Read the model definition and answer for the solid it produces. Units are mm, in the model's axes. A direction names the side the tool comes from. Round coordinates to 2 decimals unless told otherwise and drop trailing zeros. Write each loop counter-clockwise with the first axis right and the second up, starting at its lowest first coordinate (ties: lowest second). Pieces come first, ordered by that corner, then holes. Notation, with made-up numbers: (26, 78) - (36, 78) arc R28 cw to (36, 107) - close; hole circle Ø9 at (87.5, 5). An arc over 180 degrees is marked (long way). Answer as CSV lines item,"result". Start each with the question number.
1) Find section B-B on y = 0.45. State how many separate pieces and enclosed holes the cut face has, then the cut area to 3 significant figures.
2) For a pull along Z with two mould halves and no side action, classify faces 3 (the cylindrical face through (-2.216, 1.479, 4.057)), 4 (the flat face through (-5, 3, -23)), 5 (the cylindrical face through (-18.63, 1.48, -22.74)) as +Z half, -Z half, draft (parallel to the pull), parting line (faces both ways), or undercut.
3) Each of these flat-tipped pins is pushed along its axis until it touches: pin 1 (1.5 mm diameter, centred on y = 2, z = -57, fed in from +X) (3 decimals); pin 2 (0.9 mm diameter, centred on y = 1.5, z = -17.5, fed in from -X); pin 3 (1.5 mm diameter, centred on y = 2.5, z = -23, fed in from -X); pin 4 (1.8 mm diameter, centred on x = -9.95, z = -58.27, fed in from +Y). Where does it stop, or does it pass through?
4) Find section C-C on z = -35. Determine the outline of the cut face in (x, y).
5) Find section A-A on x = -5.5. Determine the outline of the cut face in (y, z).
6) Which of the six approach directions +Z, -Z, +X, -X, +Y, -Y give full straight-line access (tool end or side, diameter ignored) to faces 1 (the flat face through (-5, 0, -23)), 2 (the flat face through (-14.361, 1, -18))?
7) Consider line 1 along Z through (x, y) = (-6.75, 2.3); line 2 along Z through (x, y) = (-6.5, 2); line 3 along X through (y, z) = (1.1, -18.5). Determine where each line is inside the solid, lowest interval first.
8) Find section D-D on x = -16. Determine the outline of the cut face in (y, z), then the cut area to 3 significant figures.
Autodesk Inventor part; units mm, degrees
ref_plane "YZ Plane" through (0, 0, 0) normal (1, 0, 0) x (0, 1, 0)
ref_plane "XZ Plane" through (0, 0, 0) normal (0, 1, 0) x (-1, 0, 0)
ref_plane "XY Plane" through (0, 0, 0) normal (0, 0, 1) x (1, 0, 0)
sketch "Sketch1" plane through (0, 0, 0) normal (0, 1, 0) x (-1, 0, 0)
  arc A0 (13.7652, 13.7563) -> (-7.6488, 8.7996) centre (2.9529, 11.7331) ccw
  arc A1 (-7.6488, -55.3335) -> (13.7652, -60.2902) centre (2.9529, -58.2669) ccw
  arc A2 (-7.6723, -55.4199) -> (-7.6723, 8.8861) centre (-125.5725, -23.2669) ccw
  circle A3 centre (2.9529, 11.7331) radius 4.5
  circle A4 centre (2.9529, -58.2669) radius 4.5
  circle A5 centre (2.9529, 4.7331) radius 1
  circle A6 centre (9.9529, 11.7331) radius 1
  circle A7 centre (2.9529, 18.7331) radius 1
  circle A8 centre (-4.0471, 11.7331) radius 1
  circle A9 centre (2.9529, -65.2669) radius 1
  circle A10 centre (9.9529, -58.2669) radius 1
  circle A11 centre (2.9529, -51.2669) radius 1
  circle A12 centre (-4.0471, -58.2669) radius 1
  line L0 (14.3609, -16.1054) -> (10.3609, -16.1054)
  line L1 (10.3609, -16.1054) -> (10.3609, -19.1054)
  line L2 (10.3609, -19.1054) -> (14.3609, -19.1054)
  line L3 (14.3609, -19.1054) -> (14.3609, -16.1054)
  line L4 (14.3609, -11.7669) -> (10.3609, -14.7669) construction
  line L5 (10.3609, -11.7669) -> (14.3609, -14.7669) construction
  line L6 (0.5448, -16.1054) -> (4.5448, -16.1054)
  line L7 (4.5448, -16.1054) -> (4.5448, -19.1054)
  line L8 (4.5448, -19.1054) -> (0.5448, -19.1054)
  line L9 (0.5448, -19.1054) -> (0.5448, -16.1054)
  arc A13 (13.7652, -60.2902) -> (13.7652, 13.7563) centre (-124.6252, -23.2669) ccw
  line L10 (12.3609, -13.2669) -> (12.3609, -13.2669)
  line L11 (10.3609, -18.6054) -> (4.5448, -18.6054)
  line L12 (7.4529, -18.6054) -> (7.4529, -17.6054)
  point P0 (0, 0)
  dimension "d0" = 22
  dimension "d1" = 22
  dimension "d2" = 70
  dimension "d3" = 9
  dimension "d4" = 9
  dimension "d6" = 2
  dimension "d9" = 360
  dimension "d13" = 2
  dimension "d16" = 360
  dimension "d21" = 4
  dimension "d22" = 3
  dimension "d26" = 5.8161
  dimension "d27" = 13.8161
  dimension "d28" = 0
  dimension "d30" = 1
extrude "Extrusion1" add sketch "Sketch1" along normal blind 3
sketch "Sketch2" plane through (0, 3, 0) normal (0, 1, 0) x (1, 0, 0)
  point P0 (0, 0)
sketch "Sketch3" plane through (0, 3, 0) normal (0, 1, 0) x (1, 0, 0)
  point P0 (0, 0)
properties part number "fem"
Check values:
1,separate pieces,"1"
1,enclosed holes,"12"
1,area,"1,760 mm^2"
2,face 3,"undercut"
2,face 4,"draft"
2,face 5,"parting line"
3,pin 1,"stops at x = 8.035"
3,pin 2,"stops at x = -18.53"
3,pin 3,"stops at x = -18.63"
3,pin 4,"passes through"
4,outline,"(-18.15, 0) - (3.93, 0) - (3.93, 3) - (-18.15, 3) - close"
5,outline,"(0, -68.97) - (3, -68.97) - (3, -61.98) - (0, -61.98) - close; (0, -54.56) - (3, -54.56) - (3, 8.02) - (0, 8.02) - close; (0, 15.44) - (3, 15.44) - (3, 22.43) - (0, 22.43) - close"
6,face 1,"+Z, -Z, +X, -X, -Y"
6,face 2,"+Y, -Y"
7,line 1,"z = -68.59 to -60.68, -55.85 to 9.32, 14.15 to 22.06"
7,line 2,"z = -68.68 to -61.04, -55.5 to 8.96, 14.5 to 22.15"
7,line 3,"x = -18.55 to -14.36, -10.36 to -4.54, -0.54 to 3.46"
8,outline,"(0, -50.6) - (3, -50.6) - (3, 4.07) - (0, 4.07) - close"
8,area,"164 mm^2"
